```python
from build123d import *

# Parameters (mm, degrees)
SKETCH1_W           = 160
SKETCH1_H           = 50
SKETCH1_R           = 11.05
SKETCH1_R_2         = 2
SKETCH1_R_3         = 7.575
SKETCH1_R_4         = 6
BOSS_EXTRUDE1_DEPTH = 10


with BuildPart() as part:
    # Sketch1 → Boss-Extrude1 (new body)
    with BuildSketch(Plane(origin=(0, 0, 0), x_dir=(1, 0, 0), z_dir=(0, 1, 0))):
        Rectangle(SKETCH1_W, SKETCH1_H)
        Circle(SKETCH1_R, mode=Mode.SUBTRACT)
        with Locations((15.5, 15.5)):
            Circle(SKETCH1_R_2, mode=Mode.SUBTRACT)
        with Locations((-15.5, 15.5)):
            Circle(SKETCH1_R_2, mode=Mode.SUBTRACT)
        with Locations((-15.5, -15.5)):
            Circle(SKETCH1_R_2, mode=Mode.SUBTRACT)
        with Locations((15.5, -15.5)):
            Circle(SKETCH1_R_2, mode=Mode.SUBTRACT)
        with Locations((-67.5, 0)):
            Circle(SKETCH1_R_3, mode=Mode.SUBTRACT)
        with Locations((67.5, 0)):
            Circle(SKETCH1_R_3, mode=Mode.SUBTRACT)
        with Locations((45, 0)):
            Circle(SKETCH1_R_4, mode=Mode.SUBTRACT)
    extrude(amount=BOSS_EXTRUDE1_DEPTH)


solid = part.part
```
Design review of the part built by this model. Coordinates are the model's own, in mm. Coordinates: 2 decimals unless noted, no trailing zeros. Loops run counter-clockwise (first coordinate to the right, second up) from the corner with the lowest first, then second, coordinate; pieces in that order, holes last.
Q1. We need section C-C on z = 15.5. State the section outline as (x, y) points.
Reported:
outline: (-80, 0) - (-17.5, 0) - (-17.5, 10) - (-80, 10) - close; (-13.5, 0) - (13.5, 0) - (13.5, 10) - (-13.5, 10) - close; (17.5, 0) - (80, 0) - (80, 10) - (17.5, 10) - close
Q2. To check wall thickness, follow line 1 (X direction, y = 4, z = 0) (3 decimals); line 2 (Z direction, x = -15.5, y = 6); line 3 (X direction, y = 6, z = -15.5). State the ranges of each line that lie inside material, in increasing order.
Reported:
line 1: x = -80 to -75.075, -59.925 to -11.05, 11.05 to 39, 51 to 59.925, 75.075 to 80
line 2: z = -25 to -17.5, -13.5 to 13.5, 17.5 to 25
line 3: x = -80 to -17.5, -13.5 to 13.5, 17.5 to 80
Q3. We need section D-D on y = 6.75. State how many separate pieces and enclosed holes the cut face has, and give its area (3 significant figures).
Reported:
separate pieces: 1
enclosed holes: 8
area: 7,090 mm2
Q4. For pin 1 (15.5 mm diameter, centred on x = 45, z = 0, fed in from +Y), flat-tipped, find the tip position at first contact; note if it passes through.
Reported:
pin 1: stops at y = 10
Q5. We need section A-A on x = 7. State the section outline as (y, z) points, and give its area (3 significant figures).
Reported:
outline: (0, -25) - (10, -25) - (10, -8.55) - (0, -8.55) - close; (0, 8.55) - (10, 8.55) - (10, 25) - (0, 25) - close
area: 329 mm2
Q6. We need section B-B on z = 0. State the section outline as (x, y) points (3 decimals).
Reported:
outline: (-80, 0) - (-75.075, 0) - (-75.075, 10) - (-80, 10) - close; (-59.925, 0) - (-11.05, 0) - (-11.05, 10) - (-59.925, 10) - close; (11.05, 0) - (39, 0) - (39, 10) - (11.05, 10) - close; (51, 0) - (59.925, 0) - (59.925, 10) - (51, 10) - close; (75.075, 0) - (80, 0) - (80, 10) - (75.075, 10) - close
Q7. The part is to be moulded in two halves that separate along Z. For faces 1 (the face through (-75.068, 4.93, -0.333)), 2 (the face through (-1, 5, 25)), 3 (the face through (-80, 5, 0)), 4 (the face through (-1, 5, -25)), say which applies: +Z half, -Z half, draft (parallel to the pull), parting line (faces both ways), or undercut.
Reported:
face 1: undercut
face 2: +Z half
face 3: draft
face 4: -Z half
